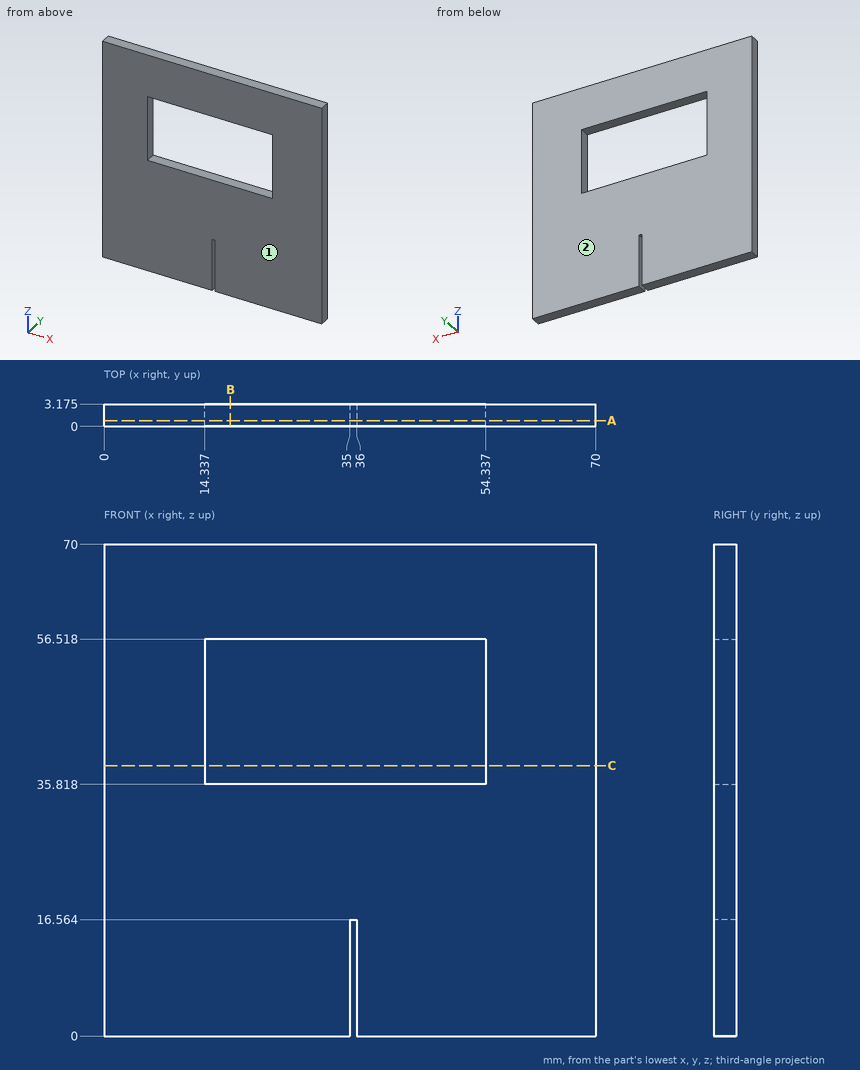
Design review of the part shown in the three views and the two pictorial views. Dimensions are in mm from the part's minimum x, y and z. Give positions to 0.01 mm unless a question says otherwise; leave off trailing zeros. Write each loop counter-clockwise with the first axis right and the second up, starting at its lowest first coordinate (ties: lowest second). Pieces come first, ordered by that corner, then holes. Notation, with made-up numbers: (34.25, 46.25) - (53.25, 46.25) arc R15 cw to (53.25, 58.25) - close; hole circle Ø9 at (-10.75, 10). An arc over 180 degrees is marked (long way). Return JSON: item names as keys, results as strings. Group by question number.
(1) To check wall thickness, follow probe 1 along X at (y, z) = (0.45, 43.5); probe 2 along Z at (x, y) = (20.5, 0.35); probe 3 along X at (y, z) = (0.75, 4). State the ranges of each line that lie inside material, in increasing order.
(2) We need section A-A, the plane y = 0.8. Give the boundary of the cut face in (x, z).
(3) Mouldability with a two-part tool opening along Y and no side actions: class the marked faces 1 and 2 as +Y half, -Y half, draft (parallel to the pull), parting line (faces both ways), or undercut.
(4) Insertion check: pin 1 (6 mm diameter, centred on x = 25, z = 54.5, fed in from -Y). The pin has a flat end and moves straight along its axis. Give the tip position at first contact, or say it passes through.
(5) We need section C-C, the plane z = 38.5. Give the boundary of the cut face in (x, y) (1 decimal).
(6) We need section B-B, the plane x = 18. Give the boundary of the cut face in (y, z) (1 decimal).
Reported:
{
 "1": {"probe 1": "x = 0 to 14.34, 54.34 to 70", "probe 2": "z = 0 to 35.82, 56.52 to 70", "probe 3": "x = 0 to 35, 36 to 70"},
 "2": {"outline": "(0, 0) - (35, 0) - (35, 16.56) - (36, 16.56) - (36, 0) - (70, 0) - (70, 70) - (0, 70) - close; hole (14.34, 35.82) - (54.34, 35.82) - (54.34, 56.52) - (14.34, 56.52) - close"},
 "3": {"face 1": "-Y half", "face 2": "+Y half"},
 "4": {"pin 1": "stops at y = 0"},
 "5": {"outline": "(0, 0) - (14.3, 0) - (14.3, 3.2) - (0, 3.2) - close; (54.3, 0) - (70, 0) - (70, 3.2) - (54.3, 3.2) - close"},
 "6": {"outline": "(0, 0) - (3.2, 0) - (3.2, 35.8) - (0, 35.8) - close; (0, 56.5) - (3.2, 56.5) - (3.2, 70) - (0, 70) - close"}
}
